Geometry: final body of the model. Coordinates: model frame, mm. Face numbers are marked on the shaded views. A direction names the side the tool comes from. Round coordinates to 2 decimals unless told otherwise and drop trailing zeros. Write each loop counter-clockwise with the first axis right and the second up, starting at its lowest first coordinate (ties: lowest second). Pieces come first, ordered by that corner, then holes. Notation, with made-up numbers: (27, 73.25) -> (38, 73.25) arc R30 cw to (38, 111.25) -> close; hole circle Ø10 at (45.25, 35.25). An arc over 180 degrees is marked (long way). Use one line per item in the form item = value. Start each with the question number.
1. Draft query along Z for the marked faces 1, 2, 3 and 4. Return one class per face: pulls with the +Z half, pulls with the -Z half, needs draft (parallel to the pull), parting line crosses it, or undercut.
2. Cut plane B-B, the plane x = -16. Return the cut outline in (y, z).
3. Cut plane A-A, the plane y = 47. Return the cut outline in (x, z), plus the area to 3 significant figures.
4. Line query: L1, parallel to Y at x = -7, z = -0.4; L2, parallel to Z at x = -9, y = 124; L3, parallel to X at y = 112, z = 21.5. Output: solid intervals per line, ascending.
5. Reachability of the marked faces 5 and 6 from +Z, -Z, +X, -X, +Y, -Y: full face, straight path, thin tool, end or side. Return the list, or none.
6. Cut plane D-D, the plane x = -25. Return the cut outline in (y, z).
7. Cut plane C-C, the plane z = 21. Return the cut outline in (x, y), plus the area to 3 significant figures.
8. Pin query (flat end, axial travel): pin 1 Ø1 at (y, z) = (59, 37) entering from +X; pin 2 Ø5 at (y, z) = (130.5, 36.5) entering from +X; pin 3 Ø10.5 at (y, z) = (116, 23.5) entering from +X. Return the tip coordinate at first contact, or that it passes through.
```python
from build123d import *

# Parameters (mm, degrees)
EXTRUDE_2_DEPTH     = 160
SKETCH_5_R          = 2.5
CUT_EXTRUDE_1_DEPTH = 169.988165266


with BuildPart() as part:
    # Sketch 4 → Extrude 2 (new body)
    with BuildSketch(Plane(origin=(0, 0, 0), x_dir=(1, 0, 0), z_dir=(0, 1, 0))):
        with BuildLine():
            Line((0, 0), (-12.5, 0))
            ThreePointArc((-12.5, 0), (-23.106601718, -4.393398282), (-27.5, -15))
            Line((-27.5, -15), (-27.5, -28))
            ThreePointArc((-27.5, -28), (-23.106601718, -38.606601718), (-12.5, -43))
            Line((-12.5, -43), (0, -43))
            Line((0, -43), (0, -44.5))
            Line((0, -44.5), (-12.5, -44.5))
            ThreePointArc((-12.5, -44.5), (-24.16726189, -39.66726189), (-29, -28))
            Line((-29, -28), (-29, -15))
            ThreePointArc((-29, -15), (-24.16726189, -3.33273811), (-12.5, 1.5))
            Line((-12.5, 1.5), (0, 1.5))
            Line((0, 1.5), (0, 0))
        make_face()
    extrude(amount=EXTRUDE_2_DEPTH)

    # Sketch 5 → Cut-Extrude 1 (cut, through all)
    with BuildSketch(Plane.XY.offset(44.5)):
        with Locations((-7, 80)):
            Circle(SKETCH_5_R)
        with Locations((-7, 47)):
            Circle(SKETCH_5_R)
        with Locations((-7, 14)):
            Circle(SKETCH_5_R)
        with Locations(Location((-7, 146, 0), (0, 0, 180))):
            Circle(SKETCH_5_R)
        with Locations(Location((-7, 113, 0), (0, 0, 180))):
            Circle(SKETCH_5_R)
    extrude(amount=-CUT_EXTRUDE_1_DEPTH, mode=Mode.SUBTRACT)


solid = part.part
```
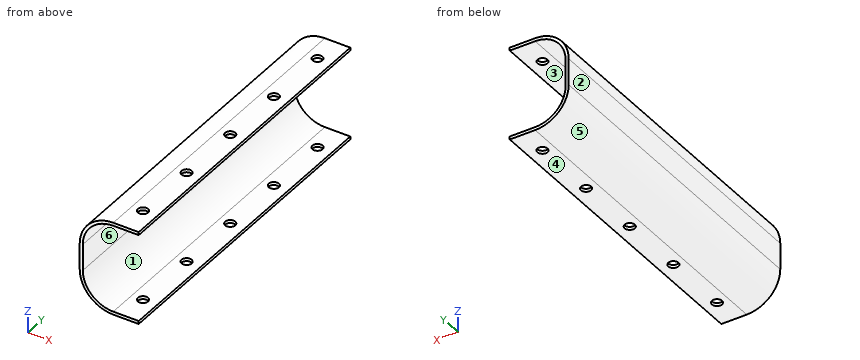
Outcome:
q1.face_1 = undercut
q1.face_2 = needs draft
q1.face_3 = undercut
q1.face_4 = pulls with the -Z half
q2.outline = (0, -1.12) -> (160, -1.12) -> (160, 0.41) -> (0, 0.41) -> close; (0, 42.59) -> (160, 42.59) -> (160, 44.12) -> (0, 44.12) -> close
q3.outline = (-29, 15) arc R16.5 ccw to (-12.5, -1.5) -> (-9.5, -1.5) -> (-9.5, 0) -> (-12.5, 0) arc R15 cw to (-27.5, 15) -> (-27.5, 28) arc R15 cw to (-12.5, 43) -> (-9.5, 43) -> (-9.5, 44.5) -> (-12.5, 44.5) arc R16.5 ccw to (-29, 28) -> close; (-4.5, -1.5) -> (0, -1.5) -> (0, 0) -> (-4.5, 0) -> close; (-4.5, 43) -> (0, 43) -> (0, 44.5) -> (-4.5, 44.5) -> close
q3.area = 116 mm^2
q4.L1 = 0 to 11.5, 16.5 to 44.5, 49.5 to 77.5, 82.5 to 110.5, 115.5 to 143.5, 148.5 to 160
q4.L2 = -1.5 to 0, 43 to 44.5
q4.L3 = -29 to -27.5
q5.face_5 = -Z, -X, +Y, -Y
q5.face_6 = +X, +Y, -Y
q6.outline = (0, 4.23) -> (160, 4.23) -> (160, 6.71) -> (0, 6.71) -> close; (0, 36.29) -> (160, 36.29) -> (160, 38.77) -> (0, 38.77) -> close
q7.outline = (-29, 0) -> (-27.5, 0) -> (-27.5, 160) -> (-29, 160) -> close
q7.area = 240 mm^2
q8.pin_1 = -24.11
q8.pin_2 = -22.7
q8.pin_3 = -27.48
